Here's how the part is built. I have some questions about the finished solid (model axes, mm). Round coordinates to 2 decimals unless told otherwise and drop trailing zeros. Order: outer loops, then holes, each group sorted by start corner. A loop starts at its lowest first (then second) coordinate and runs counter-clockwise, first axis right, second up. Notation, with made-up numbers: (25, -30.75) - (38, -30.75) arc R5 ccw to (38, -24.75) - close; hole circle Ø3 at (-11, -33.5). An arc over 180 degrees is marked (long way). Answer as a JSON object with one key per item and string values.
Solid Edge part; units mm, degrees
sketch "Sketch1" plane through (0, 0, 0) normal (0, 0, 1) x (1, 0, 0)
  circle A0 centre (0, 0) radius 39.75
extrude "ExtrudedProtrusion_1" add sketch "Sketch1" along normal mid plane 60
fillet "Round_1" radius 1 2 edges at (-39.75, 0, 30) (-39.75, 0, -30)
hole "Hole_1" at (0, 0, 30) direction (0, 0, -1) diameter 10 end up to next
fillet "Round_2" radius 1 2 edges at (-5, 0, 30) (5, 0, -30)
properties material "Acrylic, high impact grade"
1. Imagine slicing it at C-C (z = 11.5). List the corners of the cut face in (x, y) for me.
Responses:
{"outline": "circle Ø79.5 at (0, 0); hole circle Ø10 at (0, 0)"}
2. For P1, Ø2, axis at y = 6.5, z = -18, coming from the +X side; P2, Ø6, axis at y = -13.5, z = -23, coming from the -X side; P3, Ø10, axis at x = 19, z = -23.5, coming from the +Y side, each with a flat end and sliding along its axis, tell me the tip position at first contact or that it passes through.
Responses:
{"P1": "x = 39.37", "P2": "x = -38.34", "P3": "y = 37.2"}
3. If I drill on L1, parallel to Y at x = 0, z = 10; L2, parallel to Y at x = -3.5, z = -7.5; L3, parallel to X at y = -27.5, z = -25, over which ranges is the centre line in solid material (lowest first)? Write a range as [from, to].
Responses:
{"L1": "[-39.75, -5], [5, 39.75]", "L2": "[-39.6, -3.57], [3.57, 39.6]", "L3": "[-28.7, 28.7]"}
4. Imagine slicing it at A-A (y = 0). List the corners of the cut face in (x, z) for me.
Responses:
{"outline": "(-39.75, -29) arc R1 ccw to (-38.75, -30) - (-6, -30) arc R1 ccw to (-5, -29) - (-5, 29) arc R1 ccw to (-6, 30) - (-38.75, 30) arc R1 ccw to (-39.75, 29) - close; (5, -29) arc R1 ccw to (6, -30) - (38.75, -30) arc R1 ccw to (39.75, -29) - (39.75, 29) arc R1 ccw to (38.75, 30) - (6, 30) arc R1 ccw to (5, 29) - close"}
5. Thinking about a two-plate mould opening in Y: for faces 1 (the face through (-4.88, 1.08, 0.41)), 2 (the face through (-1, -8, 30)), 3 (the face through (-5.175, -39.412, -0.406)), which applies, pulls with the +Y half, pulls with the -Y half, needs draft (parallel to the pull), parting line crosses it, or undercut?
Responses:
{"face 1": "undercut", "face 2": "needs draft", "face 3": "parting line crosses it"}
